CAD build for the part. Positions are in the model's coordinates, mm. Face numbers are marked on the shaded views. A direction names the side the tool comes from. Give positions to 0.01 mm unless a question says otherwise; leave off trailing zeros. Loops run counter-clockwise (first coordinate to the right, second up) from the corner with the lowest first, then second, coordinate; pieces in that order, holes last. Notation, with made-up numbers: (16.25, -20) - (47.25, -20) arc R18 cw to (47.25, 0) - close; hole circle Ø3 at (54.5, -21). An arc over 180 degrees is marked (long way). Return JSON: item names as keys, results as strings.
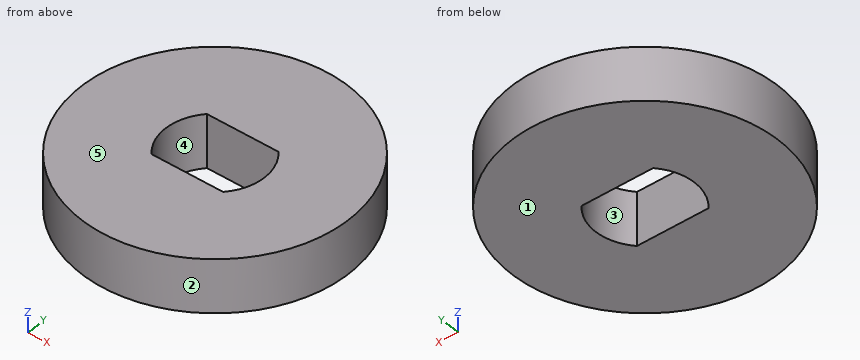
from build123d import *

# Parameters (mm, degrees)
SKETCH1_R           = 7.9375
BOSS_EXTRUDE1_DEPTH = 3.175


with BuildPart() as part:
    # Sketch1 → Boss-Extrude1 (new body)
    with BuildSketch(Plane.XY):
        Circle(SKETCH1_R)
        with BuildLine():
            ThreePointArc((-2.175224917, 1.9685), (-2.9337, 0), (-2.175224917, -1.9685))
            Line((-2.175224917, -1.9685), (2.175224917, -1.9685))
            ThreePointArc((2.175224917, -1.9685), (2.9337, 0), (2.175224917, 1.9685))
            Line((2.175224917, 1.9685), (-2.175224917, 1.9685))
        make_face(mode=Mode.SUBTRACT)
    extrude(amount=BOSS_EXTRUDE1_DEPTH)


solid = part.part
1. Which spindle directions (+Z, -Z, +X, -X, +Y, -Y) get a long thin tool onto all of the face, cutting with end or side? Do the marked faces 4 and 5. Say none if no direction does.
Values follow:
{"face 4": "+Z, -Z", "face 5": "+Z, +X, -X, +Y, -Y"}
2. Cut at B-B, the plane x = 0. Write the cut outline in (y, z) (1 decimal).
Values follow:
{"outline": "(-7.9, 0) - (-2, 0) - (-2, 3.2) - (-7.9, 3.2) - close; (2, 0) - (7.9, 0) - (7.9, 3.2) - (2, 3.2) - close"}
3. Cut at A-A, the plane y = 0. Write the cut outline in (x, z) (1 decimal), plus the area to 3 significant figures.
Values follow:
{"outline": "(-7.9, 0) - (-2.9, 0) - (-2.9, 3.2) - (-7.9, 3.2) - close; (2.9, 0) - (7.9, 0) - (7.9, 3.2) - (2.9, 3.2) - close", "area": "31.8 mm²"}
4. Drill centre lines: probe 1 along Y at (x, z) = (-2.5, 0.9); probe 2 along X at (y, z) = (-1, 1.9); probe 3 along Y at (x, z) = (-2.25, 0.35). Where is each one in solid material? Low to high.
Values follow:
{"probe 1": "y = -7.53 to -1.54, 1.54 to 7.53", "probe 2": "x = -7.87 to -2.76, 2.76 to 7.87", "probe 3": "y = -7.61 to -1.88, 1.88 to 7.61"}
5. Cut at D-D, the plane x = 5.25. Write the cut outline in (y, z) (3 decimals), plus the area to 3 significant figures.
Values follow:
{"outline": "(-5.953, 0) - (5.953, 0) - (5.953, 3.175) - (-5.953, 3.175) - close", "area": "37.8 mm²"}
6. Cut at C-C, the plane z = 1.45. Write the cut outline in (x, y) (1 decimal).
Values follow:
{"outline": "circle Ø15.9 at (0, 0); hole (-2.2, -2) - (2.2, -2) arc R2.9 ccw to (2.2, 2) - (-2.2, 2) arc R2.9 ccw to start"}
7. Pull direction X, two halves, no side cores. Call the marked faces 1, 2 and 3: +X half, -X half, draft (parallel to the pull), parting line (faces both ways), or undercut.
Values follow:
{"face 1": "draft", "face 2": "parting line", "face 3": "undercut"}
8. Drop a flat-ended pin along its axis: P1, Ø1, axis at x = -1, z = 1, coming from the -Y side. Give the stop position or say it passes through.
Values follow:
{"P1": "stops at y = -7.92"}
